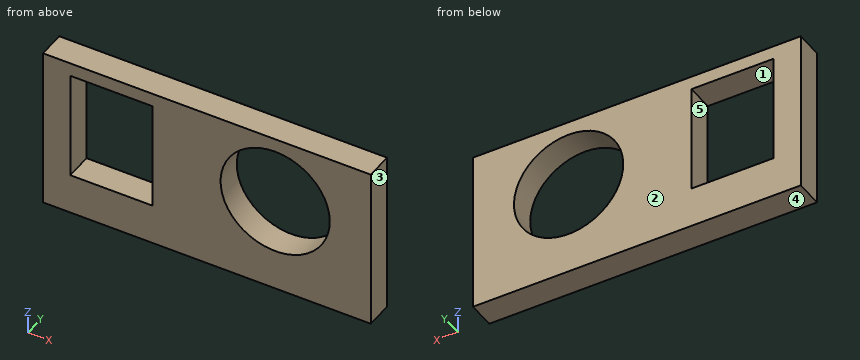
from build123d import *

# Parameters (mm, degrees)
SKIZZE1_W                       = 120
SKIZZE1_H                       = 50
AUFSATZ_LINEAR_AUSTRAGEN1_DEPTH = 10
SKIZZE3_R                       = 20
SKIZZE3_W                       = 30
SKIZZE3_H                       = 40
SCHNITT_LINEAR_AUSTRAGEN1_DEPTH = 66.76473219
SKIZZE4_W                       = 120
SKIZZE4_H                       = 10
AUFSATZ_LINEAR_AUSTRAGEN2_DEPTH = 10


with BuildPart() as part:
    # Skizze1 → Aufsatz-Linear austragen1 (new body)
    with BuildSketch(Plane(origin=(0, 0, 0), x_dir=(1, 0, 0), z_dir=(0, 1, 0))):
        Rectangle(SKIZZE1_W, SKIZZE1_H)
    extrude(amount=AUFSATZ_LINEAR_AUSTRAGEN1_DEPTH)

    # Skizze3 → Schnitt-Linear austragen1 (cut, through all)
    with BuildSketch(Plane(origin=(0, 10, 0), x_dir=(1, 0, 0), z_dir=(0, 1, 0))):
        with Locations(Location((25, 0, 0), (0, 0, 270))):
            Circle(SKIZZE3_R)
        with Locations((-35, 0)):
            Rectangle(SKIZZE3_W, SKIZZE3_H)
    extrude(amount=-SCHNITT_LINEAR_AUSTRAGEN1_DEPTH, mode=Mode.SUBTRACT)

    # Skizze4 → Aufsatz-Linear austragen2 (add)
    with BuildSketch(Plane(origin=(0, 10, 0), x_dir=(1, 0, 0), z_dir=(0, 1, 0))):
        with Locations((0, 30)):
            Rectangle(SKIZZE4_W, SKIZZE4_H)
    extrude(amount=-AUFSATZ_LINEAR_AUSTRAGEN2_DEPTH)


solid = part.part
Can you work these out from the model? Positions are in its coordinate system, mm. Face numbers are marked on the shaded views. A direction names the side the tool comes from. Round coordinates to 2 decimals unless told otherwise and drop trailing zeros. Write each loop counter-clockwise with the first axis right and the second up, starting at its lowest first coordinate (ties: lowest second). Pieces come first, ordered by that corner, then holes. Notation, with made-up numbers: M 59.5,18.25 L 65.5,18.25 A26 ccw 65.5,55.25 Z; hole C 28,14.5 d7. An arc over 180 degrees is marked long. Use a Markdown table: item, result.
Item 1: If I drill on line 1 along X through (y, z) = (2.75, 0); line 2 along Z through (x, y) = (-28.5, 6.5); line 3 along X through (y, z) = (7, 11.5), over which ranges is the centre line in solid material (lowest first)? Write a range as [from, to].
Found:
| item | result |
|---|---|
| line 1 | x = [-60, -50], [-20, 5], [45, 60] |
| line 2 | z = [-35, -20], [20, 25] |
| line 3 | x = [-60, -50], [-20, 8.64], [41.36, 60] |
Item 2: I want a section at D-D (z = 13.5). List the corners of the cut face in (x, y) for me, and give its area (3 significant figures).
Found:
| item | result |
|---|---|
| outline | M -60,0 L -50,0 L -50,10 L -60,10 Z; M -20,0 L 10.24,0 L 10.24,10 L -20,10 Z; M 39.76,0 L 60,0 L 60,10 L 39.76,10 Z |
| area | 605 mm2 |
Item 3: I want a section at A-A (z = 0). List the corners of the cut face in (x, y) for me, and give its area (3 significant figures).
Found:
| item | result |
|---|---|
| outline | M -60,0 L -50,0 L -50,10 L -60,10 Z; M -20,0 L 5,0 L 5,10 L -20,10 Z; M 45,0 L 60,0 L 60,10 L 45,10 Z |
| area | 500 mm2 |
Item 4: We'd pull the mould along X, two halves only. Please class the marked faces 1, 2 and 3: released by +X, released by -X, zero draft, split by the parting line, or undercut.
Found:
| item | result |
|---|---|
| face 1 | undercut |
| face 2 | zero draft |
| face 3 | released by +X |
Item 5: I want a section at C-C (y = 7.5). List the corners of the cut face in (x, z) for me.
Found:
| item | result |
|---|---|
| outline | M -60,-35 L 60,-35 L 60,25 L -60,25 Z; hole M -50,-20 L -20,-20 L -20,20 L -50,20 Z; hole C 25,0 d40 |
Item 6: I want a section at B-B (x = 25). List the corners of the cut face in (y, z) for me.
Found:
| item | result |
|---|---|
| outline | M 0,-35 L 10,-35 L 10,-20 L 0,-20 Z; M 0,20 L 10,20 L 10,25 L 0,25 Z |
Item 7: For pin 1 Ø1 at (x, z) = (27.5, -21.5) entering from -Y, with a flat end and sliding along its axis, tell me the tip position at first contact or that it passes through.
Found:
| item | result |
|---|---|
| pin 1 | stops at y = 0 |
Item 8: Which directions (+Z, -Z, +X, -X, +Y, -Y) give clear straight access to the entire face, cutting with the end or side of a thin tool? Please do the marked faces 4 and 5.
Found:
| item | result |
|---|---|
| face 4 | -Z, +X, -X, +Y, -Y |
| face 5 | +Y, -Y |
